Source: CAD feature listing. Evaluate the final solid. Frame: model axes, mm. A direction names the side the tool comes from. Give positions to 0.01 mm unless a question says otherwise; leave off trailing zeros. Return JSON: item names as keys, results as strings.
from build123d import *

# Parameters (mm, degrees)
SKETCH1_R           = 19.05
SKETCH1_R_2         = 6.35
SKETCH1_R_3         = 2.667
BOSS_EXTRUDE1_DEPTH = 21.59
CUT_EXTRUDE1_START  = -12.7
SKETCH2_R           = 2.667
CUT_EXTRUDE1_DEPTH  = 12.7
CUT_EXTRUDE2_DEPTH  = 42.695469184
CUT_EXTRUDE3_DEPTH  = 42.695469184


with BuildPart() as part:
    # Sketch1 → Boss-Extrude1 (new body)
    # profile 1 of 3: a face of its own
    with BuildSketch(Plane(origin=(0, 0, 0), x_dir=(1, 0, 0), z_dir=(0, 1, 0))):
        Circle(SKETCH1_R)
        with Locations(Location((0, 0, 0), (0, 0, 270))):
            Circle(SKETCH1_R_2, mode=Mode.SUBTRACT)
    # profile 2 of 3: a face of its own
    with BuildSketch(Plane(origin=(0, 0, 0), x_dir=(1, 0, 0), z_dir=(0, 1, 0))):
        with BuildLine():
            add(Edge.make_bspline(
                [(0, -19.05), (-10.097544885, -21.525800279), (-18.379445047, -27.124937251)],
                knots=[0, 0, 0, 0.663461898, 0.663461898, 0.663461898], degree=2))
            ThreePointArc((0, -19.05), (-13.470384182, -13.470384182), (-19.05, 0))
            add(Edge.make_bspline(
                [(-19.05, 0), (-21.525800279, -10.097544885), (-27.124937251, -18.379445047)],
                knots=[0, 0, 0, 0.663461898, 0.663461898, 0.663461898], degree=2))
            ThreePointArc((-27.124937251, -18.379445047), (-26.222347874, -26.222347874), (-18.379445047, -27.124937251))
        make_face()
        with Locations(Location((-21.732219813, -21.732219813, 0), (0, 0, 270))):
            Circle(SKETCH1_R_3, mode=Mode.SUBTRACT)
    # profile 3 of 3: a face of its own
    with BuildSketch(Plane(origin=(0, 0, 0), x_dir=(1, 0, 0), z_dir=(0, 1, 0))):
        with BuildLine():
            ThreePointArc((0, 19.05), (13.470384182, 13.470384182), (19.05, 0))
            add(Edge.make_bspline(
                [(19.05, 0), (21.525800279, 10.097544885), (27.124937251, 18.379445047)],
                knots=[0, 0, 0, 0.663461898, 0.663461898, 0.663461898], degree=2))
            ThreePointArc((27.124937251, 18.379445047), (26.222347874, 26.222347874), (18.379445047, 27.124937251))
            add(Edge.make_bspline(
                [(0, 19.05), (10.097544885, 21.525800279), (18.379445047, 27.124937251)],
                knots=[0, 0, 0, 0.663461898, 0.663461898, 0.663461898], degree=2))
        make_face()
        with Locations(Location((21.732219813, 21.732219813, 0), (0, 0, 270))):
            Circle(SKETCH1_R_3, mode=Mode.SUBTRACT)
    extrude(amount=BOSS_EXTRUDE1_DEPTH)

    # Sketch2 → Cut-Extrude1 (cut)
    # profile 1 of 2: a face of its own
    with BuildSketch(Plane(origin=(0, 21.59, 0), x_dir=(1, 0, 0), z_dir=(0, 1, 0)).offset(CUT_EXTRUDE1_START)):
        with BuildLine():
            add(Edge.make_bspline(
                [(-18.379445047, -27.124937251), (-10.097544885, -21.525800279), (0, -19.05)],
                knots=[0, 0, 0, 0.663461898, 0.663461898, 0.663461898], degree=2))
            ThreePointArc((0, -19.05), (-13.470384182, -13.470384182), (-19.05, 0))
            add(Edge.make_bspline(
                [(-19.05, 0), (-21.525800279, -10.097544885), (-27.124937251, -18.379445047)],
                knots=[0, 0, 0, 0.663461898, 0.663461898, 0.663461898], degree=2))
            ThreePointArc((-27.124937251, -18.379445047), (-26.222347874, -26.222347874), (-18.379445047, -27.124937251))
        make_face()
        with Locations(Location((-21.732219813, -21.732219813, 0), (0, 0, 270))):
            Circle(SKETCH2_R, mode=Mode.SUBTRACT)
    # profile 2 of 2: a face of its own
    with BuildSketch(Plane(origin=(0, 21.59, 0), x_dir=(1, 0, 0), z_dir=(0, 1, 0)).offset(CUT_EXTRUDE1_START)):
        with BuildLine():
            ThreePointArc((0, 19.05), (13.470384182, 13.470384182), (19.05, 0))
            add(Edge.make_bspline(
                [(19.05, 0), (21.525800279, 10.097544885), (27.124937251, 18.379445047)],
                knots=[0, 0, 0, 0.663461898, 0.663461898, 0.663461898], degree=2))
            ThreePointArc((27.124937251, 18.379445047), (26.222347874, 26.222347874), (18.379445047, 27.124937251))
            add(Edge.make_bspline(
                [(18.379445047, 27.124937251), (10.097544885, 21.525800279), (0, 19.05)],
                knots=[0, 0, 0, 0.663461898, 0.663461898, 0.663461898], degree=2))
        make_face()
        with Locations(Location((21.732219813, 21.732219813, 0), (0, 0, 270))):
            Circle(SKETCH2_R, mode=Mode.SUBTRACT)
    extrude(amount=CUT_EXTRUDE1_DEPTH, mode=Mode.SUBTRACT)

    # Sketch3 → Cut-Extrude2 (cut, through all)
    with BuildSketch(Plane(origin=(0, 8.89, 0), x_dir=(1, 0, 0), z_dir=(0, 1, 0))):
        with BuildLine():
            Line((24.399219813, 27.494997876), (20.006137413, 23.765327914))
            ThreePointArc((20.006137413, 23.765327914), (22.852359813, 24.152586599), (24.399219813, 21.732219813))
            ThreePointArc((24.399219813, 21.732219813), (24.152586599, 20.612079813), (23.458302213, 19.699111712))
            Line((23.458302213, 19.699111712), (27.851384613, 23.428781675))
            ThreePointArc((27.851384613, 23.428781675), (26.572953386, 25.841939813), (24.399219813, 27.494997876))
        make_face()
    extrude(amount=-CUT_EXTRUDE2_DEPTH, mode=Mode.SUBTRACT)

    # Sketch4 → Cut-Extrude3 (cut, through all)
    with BuildSketch(Plane(origin=(0, 8.89, 0), x_dir=(1, 0, 0), z_dir=(0, 1, 0))):
        with BuildLine():
            ThreePointArc((-19.699111712, -23.458302213), (-23.458302213, -23.765327914), (-23.765327914, -20.006137413))
            Line((-23.765327914, -20.006137413), (-27.494997876, -24.399219813))
            ThreePointArc((-27.494997876, -24.399219813), (-25.841939813, -26.572953386), (-23.428781675, -27.851384613))
            Line((-23.428781675, -27.851384613), (-19.699111712, -23.458302213))
        make_face()
    extrude(amount=-CUT_EXTRUDE3_DEPTH, mode=Mode.SUBTRACT)


solid = part.part
1. First-contact query: pin 1 (1.5 mm diameter, centred on x = 2.5, y = 12, fed in from -Z); pin 2 (6 mm diameter, centred on x = 14, y = 18, fed in from -Z); pin 3 (5 mm diameter, centred on x = -9.5, y = 13, fed in from -Z); pin 4 (10 mm diameter, centred on x = 0, z = 0, fed in from +Y). Flat tips, straight axial feed; report the tip coordinate or a pass-through.
Evaluation:
{"pin 1": "stops at z = -18.97", "pin 2": "stops at z = -15.55", "pin 3": "stops at z = -17.72", "pin 4": "passes through"}
2. Ray query, probe 1 along Z at (x, y) = (-2, 15); probe 2 along Y at (x, z) = (12.5, -17.5); probe 3 along X at (y, z) = (9, 3). Return the intervals inside material, ascending.
Evaluation:
{"probe 1": "z = -18.94 to -6.03, 6.03 to 18.94", "probe 2": "y = 0 to 8.89", "probe 3": "x = -18.81 to -5.6, 5.6 to 18.81"}
3. Draft query along Z for faces 6 (the face through (-17, 8.89, 17)), 7 (the face through (-19.96, 4.38, 19.74)), 8 (the face through (-28.067, 4.383, 21.299)). Return one class per face: pulls with the +Z half, pulls with the -Z half, needs draft (parallel to the pull), parting line crosses it, or undercut.
Evaluation:
{"face 6": "needs draft", "face 7": "undercut", "face 8": "parting line crosses it"}
4. Set-up query: faces 1 (the face through (-7, 0, 0)), 2 (the face through (-25.6, 4.51, 22.17)), 3 (the face through (17, 8.89, -17)), 4 (the face through (22.233, 4.507, -25.656)), 5 (the face through (25.624, 4.507, -21.538)). Return all of +Z, -Z, +X, -X, +Y, -Y with unobstructed straight access to the full face (end or side cutting, diameter ignored); none if empty.
Evaluation:
{"face 1": "+Z, -Z, +X, -X, -Y", "face 2": "+Z, +Y, -Y", "face 3": "-Z, +X, +Y", "face 4": "+X, +Y, -Y", "face 5": "+Y, -Y"}
